```python
from build123d import *


with BuildPart() as f1:
    # F0 (on Front) → F1 (revolve)
    with BuildSketch(Plane.XZ):
        with BuildLine():
            Line((17.4625, 0), (19.05, 0))
            Line((19.05, 0), (19.05, 19.05))
            Line((19.05, 19.05), (21.2725, 19.05))
            ThreePointArc((21.2725, 19.05), (23.068551, 19.793949), (23.8125, 21.59))
            Line((23.8125, 21.59), (23.8125, 101.6))
            Line((23.8125, 101.6), (23.01875, 101.6))
            Line((23.01875, 101.6), (23.01875, 22.38375))
            ThreePointArc((23.01875, 22.38375), (22.274801, 20.587699), (20.47875, 19.84375))
            Line((20.47875, 19.84375), (17.4625, 19.84375))
            Line((17.4625, 19.84375), (17.4625, 0))
        make_face()
    revolve(axis=Axis((0, 0, 3.679249), (0, 0, -1)))


solid = f1.part
```
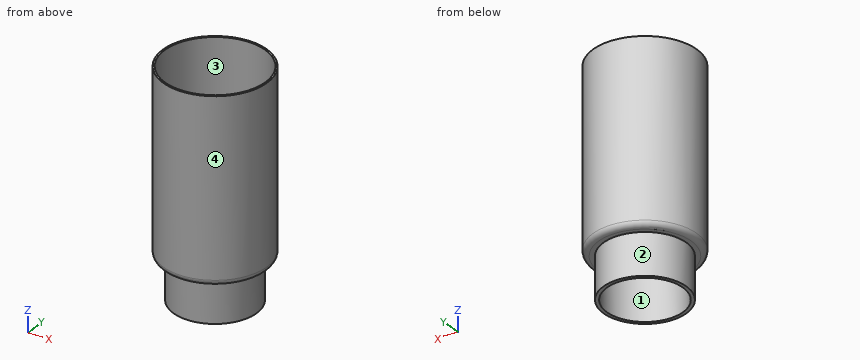
Design review of the part built by this model. Coordinates are the model's own, in mm. Face numbers are marked on the shaded views. A direction names the side the tool comes from. Coordinates: 2 decimals unless noted, no trailing zeros. Loops run counter-clockwise (first coordinate to the right, second up) from the corner with the lowest first, then second, coordinate; pieces in that order, holes last. Notation, with made-up numbers: (-0.5, 66.25) -> (26.5, 66.25) arc R11 ccw to (26.5, 74.25) -> close; hole circle Ø5 at (-14.5, -9). An arc over 180 degrees is marked (long way). Answer as a JSON object with one key per item and string values.
Q1. The part is to be moulded in two halves that separate along X. For the marked faces 1 and 2, say which applies: +X half, -X half, draft (parallel to the pull), parting line (faces both ways), or undercut.
Answer block:
{"face 1": "undercut", "face 2": "parting line"}
Q2. To check wall thickness, follow L1, parallel to Y at x = 0, z = 72; L2, parallel to X at y = 0, z = 6. State the ranges of each line that lie inside material, in increasing order.
Answer block:
{"L1": "y = -23.81 to -23.02, 23.02 to 23.81", "L2": "x = -19.05 to -17.46, 17.46 to 19.05"}
Q3. Tool access review of the marked faces 3 and 4: name each direction out of +Z, -Z, +X, -X, +Y, -Y from which nothing blocks a thin tool from reaching the whole face with its end or side.
Answer block:
{"face 3": "+Z", "face 4": "+Z, -Z"}
Q4. Clearance check with flat-ended pins moving along their axes: pin 1 Ø2 at (x, z) = (-15, 10.5) entering from -Y; pin 2 Ø2 at (y, z) = (-18, 49.5) entering from -X; pin 3 Ø8 at (y, z) = (-14.5, 47.5) entering from +X; pin 4 Ø3 at (y, z) = (-0.5, 65) entering from +X. State where each tip first meets the part, or that it passes through.
Answer block:
{"pin 1": "stops at y = -12.92", "pin 2": "stops at x = -16.67", "pin 3": "stops at x = 21.37", "pin 4": "stops at x = 23.81"}
Q5. Take a section at A-A on x = 0. Give the boundary of the cut face in (y, z), plus the area to 3 significant figures.
Answer block:
{"outline": "(-23.81, 21.59) arc R2.54 ccw to (-21.27, 19.05) -> (-19.05, 19.05) -> (-19.05, 0) -> (-17.46, 0) -> (-17.46, 19.84) -> (-20.48, 19.84) arc R2.54 cw to (-23.02, 22.38) -> (-23.02, 101.6) -> (-23.81, 101.6) -> close; (17.46, 0) -> (19.05, 0) -> (19.05, 19.05) -> (21.27, 19.05) arc R2.54 ccw to (23.81, 21.59) -> (23.81, 101.6) -> (23.02, 101.6) -> (23.02, 22.38) arc R2.54 cw to (20.48, 19.84) -> (17.46, 19.84) -> close", "area": "200 mm^2"}
Q6. Take a section at C-C on z = 56.5. Give the boundary of the cut face in (x, y) (1 decimal), plus the area to 3 significant figures.
Answer block:
{"outline": "circle Ø47.6 at (0, 0); hole circle Ø46 at (0, 0)", "area": "117 mm^2"}
